CAD build for the part. Positions are in the model's coordinates, mm. Face numbers are marked on the shaded views. A direction names the side the tool comes from. Give positions to 0.01 mm unless a question says otherwise; leave off trailing zeros. Loops run counter-clockwise (first coordinate to the right, second up) from the corner with the lowest first, then second, coordinate; pieces in that order, holes last.
Item 1: Drop flat-ended pins along their axis: P1, Ø4, axis at x = 6.5, z = 2, coming from the -Y side; P2, Ø1.5, axis at y = 37.5, z = 3, coming from the -X side; P3, Ø1.5, axis at y = 39, z = 3, coming from the +X side; P4, Ø10, axis at y = 16, z = -4, coming from the +X side. Give the stop position or say it passes through.
Item 2: Saw through at D-D on y = 49. Give the cut face in (x, z), plus the area to 3 significant figures.
Item 3: Which spindle directions (+Z, -Z, +X, -X, +Y, -Y) get a long thin tool onto all of the face, cutting with end or side? Do the marked faces 1 and 2. Say none if no direction does.
Item 4: Saw through at A-A on y = 36.5. Give the number of separate pieces and of enclosed holes in the cut face, plus the area to 3 significant figures.
Item 5: Probe probe 1 along Y at (x, z) = (65, 1); probe 2 along Z at (x, y) = (48.5, 34.5); probe 3 along X at (y, z) = (36, 1). List the from-to ranges inside material, lowest first.
Item 6: Saw through at C-C on y = 63.5. Give the cut face in (x, z), plus the area to 3 significant figures.
Item 7: Saw through at B-B on x = 65. Give the cut face in (y, z).
Item 8: Mould opens along X. For the marked faces 3, 4, 5 and 6 say: released by +X, released by -X, zero draft, split by the parting line, or undercut.
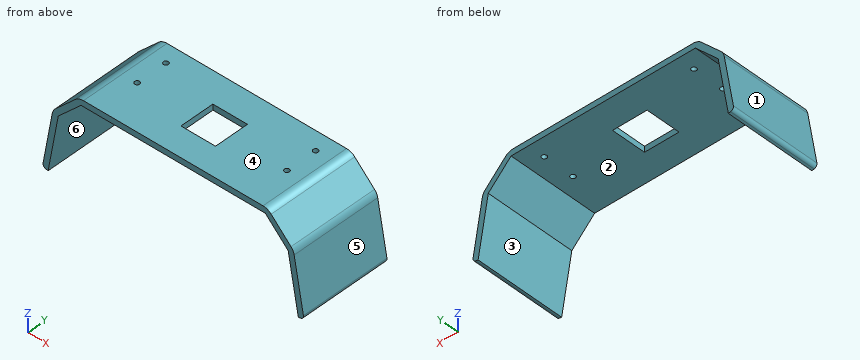
from build123d import *

# Parameters (mm, degrees)
BOSS_EXTRUDE1_DEPTH = 78.5
FILLET1_R           = 10
FILLET2_R           = 10
FILLET12_R          = 10
FILLET13_R          = 3
SKETCH2_W           = 30
SKETCH2_H           = 30
CUT_EXTRUDE1_DEPTH  = 78.5
SKETCH4_R           = 2.15
CUT_EXTRUDE2_DEPTH  = 78.5


with BuildPart() as part:
    # Sketch1 → Boss-Extrude1 (new body)
    with BuildSketch(Plane(origin=(0, 0, 0), x_dir=(1, 0, 0), z_dir=(0, 1, 0))):
        Polygon((-80, 0), (80, 0), (99.798989873, 19.798989873), (108.615338909, 69.798989873), (113.539377674, 68.930748985), (104.449273338, 17.378205526), (82.071067812, -5), (-82.071067812, -5), (-104.449273338, 17.378205526), (-113.539377674, 68.930748985), (-108.615338909, 69.798989873), (-99.798989873, 19.798989873), align=None)
    extrude(amount=BOSS_EXTRUDE1_DEPTH)

    # Fillet1
    fillet1_edges = [part.edges().sort_by_distance(p)[0] for p in [
        (82.071067812, 39.25, 5),
    ]]
    fillet(fillet1_edges, radius=FILLET1_R)

    # Fillet2
    fillet2_edges = [part.edges().sort_by_distance(p)[0] for p in [
        (104.449273338, 39.25, -17.378205526),
    ]]
    fillet(fillet2_edges, radius=FILLET2_R)

    # Fillet12
    fillet12_edges = [part.edges().sort_by_distance(p)[0] for p in [
        (-104.449273338, 39.25, -17.378205526),
        (-82.071067812, 39.25, 5),
    ]]
    fillet(fillet12_edges, radius=FILLET12_R)

    # Fillet13
    fillet13_edges = [part.edges().sort_by_distance(p)[0] for p in [
        (-113.539377674, 39.25, -68.930748985),
        (113.539377674, 39.25, -68.930748985),
    ]]
    fillet(fillet13_edges, radius=FILLET13_R)

    # Sketch2 → Cut-Extrude1 (cut)
    with BuildSketch(Plane.XY.offset(5)):
        with Locations((0, 38.5)):
            Rectangle(SKETCH2_W, SKETCH2_H)
    extrude(amount=-CUT_EXTRUDE1_DEPTH, mode=Mode.SUBTRACT)

    # Sketch4 → Cut-Extrude2 (cut)
    with BuildSketch(Plane.XY.offset(5)):
        with Locations((65, 36.5)):
            Circle(SKETCH4_R)
        with Locations((65, 63.5)):
            Circle(SKETCH4_R)
        with Locations((-65, 63.5)):
            Circle(SKETCH4_R)
        with Locations((-65, 36.5)):
            Circle(SKETCH4_R)
    extrude(amount=-CUT_EXTRUDE2_DEPTH, mode=Mode.SUBTRACT)


solid = part.part
Results below:
1. P1: stops at y = 0
1. P2: stops at x = -84.82
1. P3: stops at x = 84.82
1. P4: stops at x = 96.07
2. outline: (-113.02, -65.98) arc R3 ccw to (-110.58, -69.45) - (-108.62, -69.8) - (-99.8, -19.8) - (-80, 0) - (-15, 0) - (-15, 5) - (-77.93, 5) arc R10 ccw to (-85, 2.07) - (-102.22, -15.15) arc R10 ccw to (-105, -20.48) - close; (15, 0) - (80, 0) - (99.8, -19.8) - (108.62, -69.8) - (110.58, -69.45) arc R3 ccw to (113.02, -65.98) - (105, -20.48) arc R10 ccw to (102.22, -15.15) - (85, 2.07) arc R10 ccw to (77.93, 5) - (15, 5) - close
2. area: 1,460 mm2
3. face 1: +Z, -X, +Y, -Y
3. face 2: -Z, +Y, -Y
4. separate pieces: 4
4. enclosed holes: 0
4. area: 1,420 mm2
5. probe 1: y = 0 to 34.35, 38.65 to 61.35, 65.65 to 78.5
5. probe 2: z = 0 to 5
5. probe 3: x = -86.07 to -67.09, -62.91 to -15, 15 to 62.91, 67.09 to 86.07
6. outline: (-113.02, -65.98) arc R3 ccw to (-110.58, -69.45) - (-108.62, -69.8) - (-99.8, -19.8) - (-80, 0) - (-67.15, 0) - (-67.15, 5) - (-77.93, 5) arc R10 ccw to (-85, 2.07) - (-102.22, -15.15) arc R10 ccw to (-105, -20.48) - close; (-62.85, 0) - (62.85, 0) - (62.85, 5) - (-62.85, 5) - close; (67.15, 0) - (80, 0) - (99.8, -19.8) - (108.62, -69.8) - (110.58, -69.45) arc R3 ccw to (113.02, -65.98) - (105, -20.48) arc R10 ccw to (102.22, -15.15) - (85, 2.07) arc R10 ccw to (77.93, 5) - (67.15, 5) - close
6. area: 1,570 mm2
7. outline: (0, 0) - (34.35, 0) - (34.35, 5) - (0, 5) - close; (38.65, 0) - (61.35, 0) - (61.35, 5) - (38.65, 5) - close; (65.65, 0) - (78.5, 0) - (78.5, 5) - (65.65, 5) - close
8. face 3: undercut
8. face 4: zero draft
8. face 5: released by +X
8. face 6: undercut
